```python
from build123d import *

# Parameters (mm, degrees)
SKETCH_W        = 45
SKETCH_H        = 15
SKETCH_R        = 3.1
PAD_DEPTH       = 8.5
POCKET_DEPTH    = 5
SKETCH002_R     = 6.45
POCKET001_DEPTH = 3
FILLET_R        = 6


with BuildPart() as part:
    # Sketch → Pad (new body)
    with BuildSketch(Plane.XY):
        Rectangle(SKETCH_W, SKETCH_H)
        Circle(SKETCH_R, mode=Mode.SUBTRACT)
    extrude(amount=PAD_DEPTH)

    # Sketch001 → Pocket (cut)
    with BuildSketch(Plane.XY.offset(8.5)):
        Polygon((3.025, -5.239454), (6.05, 0), (3.025, 5.239454), (-3.025, 5.239454), (-6.05, 0), (-3.025, -5.239454), align=None)
    extrude(amount=-POCKET_DEPTH, mode=Mode.SUBTRACT)

    # Sketch002 → Pocket001 (cut)
    with BuildSketch(Plane.XY.offset(8.5)):
        with Locations((15, 0)):
            Circle(SKETCH002_R)
        with Locations((-15, 0)):
            Circle(SKETCH002_R)
    extrude(amount=-POCKET001_DEPTH, mode=Mode.SUBTRACT)

    # Fillet
    fillet_edges = [part.edges().sort_by_distance(p)[0] for p in [
        (-22.5, -7.5, 4.25),
        (-22.5, 7.5, 4.25),
        (22.5, 7.5, 4.25),
        (22.5, -7.5, 4.25),
    ]]
    fillet(fillet_edges, radius=FILLET_R)


solid = part.part
```
Part model, mm, in its own coordinate system. A direction names the side the tool comes from. Round coordinates to 2 decimals unless told otherwise and drop trailing zeros. Order: outer loops, then holes, each group sorted by start corner. A loop starts at its lowest first (then second) coordinate and runs counter-clockwise, first axis right, second up. Notation, with made-up numbers: M -15,17.25 L 19,17.25 A20 cw 19,35.25 Z; hole C -38,-3.75 d2. An arc over 180 degrees is marked long. Put each result on its own line as item: value. Start each with the question number.
1. Tool access for faces 4 (the face through (-20.789, -5.696, 4.31)), 5 (the face through (-4.56, -2.58, 6.04)): list every direction of +Z, -Z, +X, -X, +Y, -Y with a clear straight run to the whole face (end or side of a thin tool).
2. Drill centre lines: probe 1 along X at (y, z) = (0, 2.55); probe 2 along X at (y, z) = (-3.25, 7); probe 3 along Y at (x, z) = (-2, 4.25). Where is each one in solid material? Low to high. Write a range as [from, to].
3. Two-plate mould, pull along X, no slides. Class faces 1 (the face through (-0.3, 3.4, 0)), 2 (the face through (4.56, 2.58, 6.04)), 3 (the face through (20.696, 5.789, 4.31)): +X half, -X half, draft (parallel to the pull), parting line (faces both ways), or undercut.
4. Slice it at C-C on y = 2.25. List the corners of the cut face in (x, z).
5. Slice it at B-B on z = 7.25. List the corners of the cut face in (x, y) (3 decimals).
6. Slice it at A-A on x = 0. List the corners of the cut face in (y, z), then the cut area to 3 significant figures.
7. Slice it at D-D on x = 15. List the corners of the cut face in (y, z).
Findings:
1. face 4: +Z, -Z, -X, -Y
1. face 5: +Z
2. probe 1: [-22.5, -3.1], [3.1, 22.5]
2. probe 2: [-22.24, -20.57], [-9.43, -4.17], [4.17, 9.43], [20.57, 22.24]
2. probe 3: [-7.5, -5.24], [5.24, 7.5]
3. face 1: draft
3. face 2: undercut
3. face 3: +X half
4. outline: M -22.45,0 L -2.13,0 L -2.13,3.5 L -4.75,3.5 L -4.75,8.5 L -8.96,8.5 L -8.96,5.5 L -21.04,5.5 L -21.04,8.5 L -22.45,8.5 Z; M 2.13,0 L 22.45,0 L 22.45,8.5 L 21.04,8.5 L 21.04,5.5 L 8.96,5.5 L 8.96,8.5 L 4.75,8.5 L 4.75,3.5 L 2.13,3.5 Z
5. outline: M -22.5,-1.5 A6 ccw -16.5,-7.5 L 16.5,-7.5 A6 ccw 22.5,-1.5 L 22.5,1.5 A6 ccw 16.5,7.5 L -16.5,7.5 A6 ccw -22.5,1.5 Z; hole C -15,0 d12.9; hole M -6.05,0 L -3.025,-5.239 L 3.025,-5.239 L 6.05,0 L 3.025,5.239 L -3.025,5.239 Z; hole C 15,0 d12.9
6. outline: M -7.5,0 L -3.1,0 L -3.1,3.5 L -5.24,3.5 L -5.24,8.5 L -7.5,8.5 Z; M 3.1,0 L 7.5,0 L 7.5,8.5 L 5.24,8.5 L 5.24,3.5 L 3.1,3.5 Z
6. area: 53.4 mm2
7. outline: M -7.5,0 L 7.5,0 L 7.5,8.5 L 6.45,8.5 L 6.45,5.5 L -6.45,5.5 L -6.45,8.5 L -7.5,8.5 Z
